from build123d import *

# Parameters (mm, degrees)
SKETCH_W      = 57.5
SKETCH_H      = 57.5
PAD_DEPTH     = 3
SKETCH001_W   = 57.5
SKETCH001_H   = 57.5
SKETCH001_W_2 = 51.5
SKETCH001_H_2 = 51.5
PAD001_DEPTH  = 3
SKETCH002_W   = 57.5
SKETCH002_H   = 57.5
SKETCH002_W_2 = 54.5
SKETCH002_H_2 = 54.5
PAD002_DEPTH  = 3
SKETCH003_W   = 10
SKETCH003_H   = 6
POCKET_DEPTH  = 5
FILLET_R      = 3


with BuildPart() as part:
    # Sketch → Pad (new body)
    with BuildSketch(Plane.XY):
        Rectangle(SKETCH_W, SKETCH_H)
    extrude(amount=PAD_DEPTH)

    # Sketch001 (on Face6 of Pad) → Pad001 (join)
    with BuildSketch(Plane.XY.offset(3)):
        Rectangle(SKETCH001_W, SKETCH001_H)
        Rectangle(SKETCH001_W_2, SKETCH001_H_2, mode=Mode.SUBTRACT)
    extrude(amount=PAD001_DEPTH)

    # Sketch002 (on Face9 of Pad001) → Pad002 (join)
    with BuildSketch(Plane.XY.offset(6)):
        Rectangle(SKETCH002_W, SKETCH002_H)
        Rectangle(SKETCH002_W_2, SKETCH002_H_2, mode=Mode.SUBTRACT)
    extrude(amount=PAD002_DEPTH)

    # Sketch003 (on Face10 of Pad002) → Pocket (cut)
    with BuildSketch(Plane.XZ.offset(28.75)):
        with Locations((0, 6)):
            Rectangle(SKETCH003_W, SKETCH003_H)
    extrude(amount=-POCKET_DEPTH, mode=Mode.SUBTRACT)

    # Fillet
    fillet_edges = [part.edges().sort_by_distance(p)[0] for p in [
        (-28.75, -28.75, 7.5),
        (-28.75, -28.75, 4.5),
        (-28.75, -28.75, 1.5),
        (-28.75, 28.75, 7.5),
        (-28.75, 28.75, 4.5),
        (-28.75, 28.75, 1.5),
        (28.75, -28.75, 7.5),
        (28.75, -28.75, 4.5),
        (28.75, -28.75, 1.5),
        (28.75, 28.75, 1.5),
        (28.75, 28.75, 4.5),
        (28.75, 28.75, 7.5),
    ]]
    fillet(fillet_edges, radius=FILLET_R)


solid = part.part
Could you check a few things on this model? Use its own coordinates, in mm. A direction names the side the tool comes from. Coordinates: 2 decimals unless noted, no trailing zeros. Loops run counter-clockwise (first coordinate to the right, second up) from the corner with the lowest first, then second, coordinate; pieces in that order, holes last.
1. For faces 1 (the face through (27.85, 27.89, 4.44)), 2 (the face through (5, -28, 5)), 3 (the face through (-27.25, 0, 7)), which set-ups out of +Z, -Z, +X, -X, +Y, -Y let a thin tool reach every point of the face, with its end or its side?
2. Imagine slicing it at B-B (z = 4.25). Please give me the cut outline in (x, y), and give its area (3 significant figures).
3. We'd pull the mould along X, two halves only. Please class faces 4 (the face through (-27.89, 27.85, 4.44)), 5 (the face through (0, 26, 6)), 6 (the face through (0, 28, 9)): released by +X, released by -X, zero draft, split by the parting line, or undercut.
4. Imagine slicing it at A-A (x = -9). Please give me the cut outline in (y, z).
5. For P1, Ø15.5, axis at x = -4.5, y = 0.5, coming from the +Z side; P2, Ø2.5, axis at y = -27.5, z = 5.5, coming from the -X side; P3, Ø0.9, axis at y = -26.5, z = 6.5, coming from the +X side, each with a flat end and sliding along its axis, tell me the tip position at first contact or that it passes through.
6. Imagine slicing it at D-D (x = -2). Please give me the cut outline in (y, z).
7. I need wall thicknesses on L1, parallel to X at y = -14, z = 4; L2, parallel to X at y = -7, z = 8. Which ranges of each line are inside material? Lowest first, please.
Computed values:
1. face 1: +Z, -Z, +X, +Y
1. face 2: +Z, -Y
1. face 3: +Z
2. outline: (-28.75, -25.75) arc R3 ccw to (-25.75, -28.75) - (-5, -28.75) - (-5, -25.75) - (-25.75, -25.75) - (-25.75, 25.75) - (25.75, 25.75) - (25.75, -25.75) - (5, -25.75) - (5, -28.75) - (25.75, -28.75) arc R3 ccw to (28.75, -25.75) - (28.75, 25.75) arc R3 ccw to (25.75, 28.75) - (-25.75, 28.75) arc R3 ccw to (-28.75, 25.75) - close
2. area: 616 mm2
3. face 4: released by -X
3. face 5: undercut
3. face 6: zero draft
4. outline: (-28.75, 0) - (28.75, 0) - (28.75, 9) - (27.25, 9) - (27.25, 6) - (25.75, 6) - (25.75, 3) - (-25.75, 3) - (-25.75, 6) - (-27.25, 6) - (-27.25, 9) - (-28.75, 9) - close
5. P1: stops at z = 3
5. P2: stops at x = -28.71
5. P3: stops at x = 28.73
6. outline: (-28.75, 0) - (28.75, 0) - (28.75, 9) - (27.25, 9) - (27.25, 6) - (25.75, 6) - (25.75, 3) - (-28.75, 3) - close
7. L1: x = -28.75 to -25.75, 25.75 to 28.75
7. L2: x = -28.75 to -27.25, 27.25 to 28.75
